from build123d import *

# Parameters (mm, degrees)
SKETCH1_W                       = 165.1
SKETCH1_H                       = 114.3
BOSS_EXTRUDE1_DEPTH             = 3.175
SKETCH3_R                       = 3.96875
CUT_EXTRUDE2_DEPTH              = 1.5875
F_6_32_TAPPED_HOLE1_D           = 2.7051
SKETCH11_W                      = 107.95
SKETCH11_H                      = 71.12
SKETCH11_W_2                    = 6.35
CUT_EXTRUDE3_DEPTH              = 101.452504324
FILLET1_R                       = 3.175
F_27_0_144_DIAMETER_HOLE1_D     = 3.6576
F_27_0_144_DIAMETER_HOLE1_DEPTH = 3.302
F_27_0_144_DIAMETER_HOLE1_TIP   = 1.0988539


with BuildPart() as part:
    # Sketch1 → Boss-Extrude1 (new body)
    with BuildSketch(Plane(origin=(0, 0, 0), x_dir=(1, 0, 0), z_dir=(0, 1, 0))):
        Rectangle(SKETCH1_W, SKETCH1_H)
    extrude(amount=BOSS_EXTRUDE1_DEPTH)

    # Sketch3 → Cut-Extrude2 (cut)
    with BuildSketch(Plane(origin=(0, 3.175, 0), x_dir=(1, 0, 0), z_dir=(0, 1, 0))):
        with Locations(Location((-73.025, 47.625, 0), (0, 0, 270))):
            Circle(SKETCH3_R)
        with Locations(Location((-73.025, -47.625, 0), (0, 0, 270))):
            Circle(SKETCH3_R)
        with Locations(Location((73.025, 47.625, 0), (0, 0, 270))):
            Circle(SKETCH3_R)
        with Locations(Location((73.025, -47.625, 0), (0, 0, 270))):
            Circle(SKETCH3_R)
    extrude(amount=-CUT_EXTRUDE2_DEPTH, mode=Mode.SUBTRACT)

    # #6-32 Tapped Hole1 (through all)
    with Locations(Plane(origin=(0, 3.175, 0), x_dir=(-1, 0, 0), z_dir=(0, 1, 0))):
        with Locations((50.8, -44.45), (-50.8, -44.45), (-50.8, 44.45), (50.8, 44.45)):
            Hole(F_6_32_TAPPED_HOLE1_D / 2)

    # Sketch11 → Cut-Extrude3 (cut, through all)
    with BuildSketch(Plane(origin=(0, 3.175, 0), x_dir=(1, 0, 0), z_dir=(0, 1, 0))):
        Rectangle(SKETCH11_W, SKETCH11_H)
        with Locations((57.15, 0)):
            Rectangle(SKETCH11_W_2, SKETCH11_H)
    extrude(amount=-CUT_EXTRUDE3_DEPTH, mode=Mode.SUBTRACT)

    # Fillet1
    fillet1_edges = [part.edges().sort_by_distance(p)[0] for p in [
        (60.325, 1.5875, 35.56),
        (-53.975, 1.5875, 35.56),
        (-53.975, 1.5875, -35.56),
        (60.325, 1.5875, -35.56),
    ]]
    fillet(fillet1_edges, radius=FILLET1_R)

    # #27 (0.144) Diameter Hole1
    with Locations(Plane(origin=(0, 3.175, 0), x_dir=(-1, 0, 0), z_dir=(0, 1, 0))):
        with Locations((73.025, -38.1), (73.025, 38.1), (-73.025, -38.1), (-73.025, 38.1)):
            Hole(F_27_0_144_DIAMETER_HOLE1_D / 2, depth=F_27_0_144_DIAMETER_HOLE1_DEPTH)
            with Locations((0, 0, -(F_27_0_144_DIAMETER_HOLE1_DEPTH + F_27_0_144_DIAMETER_HOLE1_TIP / 2))):  # 118° drill point
                Cone(0, F_27_0_144_DIAMETER_HOLE1_D / 2, F_27_0_144_DIAMETER_HOLE1_TIP, mode=Mode.SUBTRACT)


solid = part.part
The model under review builds one solid part; all positions refer to its coordinate system, in mm. A direction names the side the tool comes from. Coordinates: 2 decimals unless noted, no trailing zeros. Write each loop counter-clockwise with the first axis right and the second up, starting at its lowest first coordinate (ties: lowest second). Pieces come first, ordered by that corner, then holes. Notation, with made-up numbers: (15, 78.25) - (58, 78.25) arc R28 cw to (58, 103.25) - close; hole circle Ø4 at (49.5, 0). An arc over 180 degrees is marked (long way). Answer as CSV lines item,"result".
(1) Clearance check with a flat-ended pin moving along its axis: pin 1 Ø4 at (x, z) = (73, -49) entering from +Y. State where the tip first meets the part, or that it passes through.
Data:
pin 1,"stops at y = 1.59"
(2) Mouldability with a two-part tool opening along X and no side actions: class faces 4 (the flat face through (-1, 2, 57.15)), 5 (the flat face through (82.55, 2, 1)), 6 (the cylindrical face through (-53.02, 1.565, 34.655)), 7 (the flat face through (-53.975, 2, 0)) as pulls with the +X half, pulls with the -X half, needs draft (parallel to the pull), parting line crosses it, or undercut.
Data:
face 4,"needs draft"
face 5,"pulls with the +X half"
face 6,"undercut"
face 7,"undercut"
(3) For line 1 along Z through (x, y) = (50.8, 1.95); line 2 along X through (y, z) = (2.5, 8.5) (3 decimals); line 3 along Z through (x, y) = (8, 1.05), list the stretches that pass through material, from the lowest coordinate up. Write a range as [from, to].
Data:
line 1,"z = [-57.15, -45.8], [-43.1, -35.56], [35.56, 43.1], [45.8, 57.15]"
line 2,"x = [-82.55, -53.975], [60.325, 82.55]"
line 3,"z = [-57.15, -35.56], [35.56, 57.15]"
(4) We need section C-C (z = -38.1). Give the boundary of the cut face in (x, y) (3 decimals).
Data:
outline,"(-82.55, 0) - (-74.854, 0) - (-74.854, 3.175) - (-82.55, 3.175) - close; (-71.196, 0) - (71.196, 0) - (71.196, 3.175) - (-71.196, 3.175) - close; (74.854, 0) - (82.55, 0) - (82.55, 3.175) - (74.854, 3.175) - close"
(5) We need section D-D (y = 0.65). Count the separate pieces of the cut face and the enclosed holes in it, plus the area to 3 significant figures.
Data:
separate pieces,"1"
enclosed holes,"9"
area,"10,700 mm2"
(6) Tool access review of faces 1 (the flat face through (-82.55, 2, 1)), 2 (the flat face through (-73, 1.588, 48)), 3 (the flat face through (2, 2, 35.56)): name each direction out of +Z, -Z, +X, -X, +Y, -Y from which nothing blocks a thin tool from reaching the whole face with its end or side.
Data:
face 1,"+Z, -Z, -X, +Y, -Y"
face 2,"+Y"
face 3,"+Y, -Y"
(7) We need section A-A (x = -40). Give the boundary of the cut face in (y, z) (3 decimals), plus the area to 3 significant figures.
Data:
outline,"(0, -57.15) - (3.175, -57.15) - (3.175, -35.56) - (0, -35.56) - close; (0, 35.56) - (3.175, 35.56) - (3.175, 57.15) - (0, 57.15) - close"
area,"137 mm2"
(8) We need section B-B (z = 6). Give the boundary of the cut face in (x, y) (3 decimals), plus the area to 3 significant figures.
Data:
outline,"(-82.55, 0) - (-53.975, 0) - (-53.975, 3.175) - (-82.55, 3.175) - close; (60.325, 0) - (82.55, 0) - (82.55, 3.175) - (60.325, 3.175) - close"
area,"161 mm2"
